The listing builds one solid part. Answer for the finished solid, in the listing's coordinates (mm). A direction names the side the tool comes from. Coordinates: 2 decimals unless noted, no trailing zeros. Loops run counter-clockwise (first coordinate to the right, second up) from the corner with the lowest first, then second, coordinate; pieces in that order, holes last. Notation, with made-up numbers: (-32.75, 86.5) - (-4.75, 86.5) arc R18 cw to (-4.75, 99.5) - close; hole circle Ø9 at (-30.75, -28.75). An arc over 180 degrees is marked (long way). Write each question's results on one line, items separated by ' | '. Start each with the question number.
(1) Find section B-B on z = 11.25. Determine the outline of the cut face in (x, y), then the cut area to 3 significant figures.
(2) Find section A-A on y = 3. Determine the outline of the cut face in (x, z), then the cut area to 3 significant figures.
(3) Find section D-D on x = -19. Determine the outline of the cut face in (y, z), then the cut area to 3 significant figures.
(4) Given pin 1 Ø1.5 at (x, y) = (-1, 2) entering from -Z; pin 2 Ø1.8 at (y, z) = (3.5, 7.5) entering from +X; pin 3 Ø3 at (y, z) = (1.5, 10.5) entering from -X; pin 4 Ø1.8 at (y, z) = (3, 3.1) entering from +X, each flat-ended and moving along its own axis, determine where each tip first touches the part or whether it passes through.
(5) Consider line 1 (Y direction, x = -18.5, z = 3.1); line 2 (Z direction, x = -1.5, y = 3.9); line 3 (X direction, y = 5.05, z = 5.5). Determine where each line is inside the solid, lowest interval first. Write a range as from..to.
(6) For faces 4 (the flat face through (-6.1, 3, 6)), 5 (the flat face through (-11, 0, 10)), 6 (the flat face through (-2, 3, 9)), determine the directions among +Z, -Z, +X, -X, +Y, -Y from which every point of the face is accessible in a straight line to the end or side of a thin tool.
(7) Determine the mould class of faces 1 (the flat face through (-5, 3, 17)), 2 (the flat face through (-3, 3, 11)), 3 (the flat face through (0, 3, 13)) for opening direction X: released by +X, released by -X, zero draft, split by the parting line, or undercut.
(8) Find section C-C on x = -5. Determine the outline of the cut face in (y, z).
Autodesk Inventor part; units mm, degrees
ref_plane "YZ Plane" through (0, 0, 0) normal (1, 0, 0) x (0, 1, 0)
ref_plane "XZ Plane" through (0, 0, 0) normal (0, 1, 0) x (-1, 0, 0)
ref_plane "XY Plane" through (0, 0, 0) normal (0, 0, 1) x (1, 0, 0)
sketch "Sketch1" plane through (0, 0, 0) normal (0, 1, 0) x (-1, 0, 0)
  line L0 (0, 0) -> (21.6, 0)
  line L1 (21.6, 0) -> (21.6, 17)
  line L2 (21.6, 17) -> (0, 17)
  line L3 (0, 17) -> (0, 0)
  line L4 (6.1, 13) -> (3, 13)
  line L5 (3, 13) -> (3, 0)
  line L6 (3, 0) -> (6.1, 0)
  line L7 (6.1, 0) -> (6.1, 13)
  line L8 (21.6, 17) -> (9.1, 17)
  line L9 (9.1, 17) -> (9.1, 0)
  line L10 (9.1, 0) -> (21.6, 0)
  line L11 (21.6, 0) -> (21.6, 17)
  line L12 (9.1, 17) -> (21.6, 6.2)
  point P0 (21.6, 6.2)
  point P1 (9.1, 17)
  dimension "d1" = 17
  dimension "d2" = 3.1
  dimension "d3" = 3
  dimension "d4" = 3
  dimension "d5" = 6.2
  dimension "d17" = 13
  dimension "d18" = 12.5
extrude "Extrusion1" add sketch "Sketch1" along normal blind 6 contours L3 L2 L9 L0 L7 L4 L5 | L12 L1 L0 L9
sketch "Sketch2" plane through (-21.6, 0, 0) normal (-1, 0, 0) x (0, 0, 1)
  circle A0 centre (3.1, 3) radius 3
  line L0 (0, 0) -> (13, 0)
  line L1 (0, 0) -> (0, 6)
  line L2 (17, 6) -> (0, 6)
  line L3 (0, 0) -> (6.2302, 0)
  line L4 (6.2302, 0) -> (6.2302, 6)
  line L5 (6.2302, 6) -> (0, 6)
  line L6 (0, 6) -> (0, 0)
  circle A1 centre (3.1, 3) radius 1
  point P0 (3.1, 6)
  point P1 (3.1, 0)
  dimension "d8" = 3.1
  dimension "d9" = 2
extrude "Extrusion2" cut sketch "Sketch2" against normal up to surface (18.6 mm away) contours A0 L0 L1 L2 | A1
sketch "Sketch3" plane through (0, 6, 0) normal (0, 1, 0) x (1, 0, 0)
  line L0 (-3, 0) -> (-3, -13)
  line L1 (0, 0) -> (-3, 0)
  line L2 (-3, -9) -> (0, -9)
  line L3 (0, -9) -> (0, 0)
  line L4 (0, 0) -> (-3, 0)
  line L5 (-3, 0) -> (-3, -9)
  line L6 (-3, -13) -> (-6.1, -13)
  line L7 (-9.1, -17) -> (0, -17)
  dimension "d13" = 8
extrude "Extrusion3" cut sketch "Sketch3" against normal blind 10
properties part number "Pi3B_spacer_R"
Values:
1) outline: (-15.76, 0) - (-6.1, 0) - (-6.1, 6) - (-15.76, 6) - close; (-3, 0) - (0, 0) - (0, 6) - (-3, 6) - close | area: 75.9 mm²
2) outline: (-21.6, 0.1) - (-6.1, 0.1) - (-6.1, 2.1) - (-21.6, 2.1) - close; (-21.6, 4.1) - (-6.1, 4.1) - (-6.1, 13) - (-3, 13) - (-3, 9) - (0, 9) - (0, 17) - (-9.1, 17) - (-21.6, 6.2) - close | area: 200 mm²
3) outline: (0, 3.1) arc R3 ccw to (6, 3.1) - (6, 8.45) - (0, 8.45) - close; hole circle Ø2 at (3, 3.1) | area: 43.1 mm²
4) pin 1: stops at z = 9 | pin 2: stops at x = -6.1 | pin 3: stops at x = -18.36 | pin 4: passes through
5) line 1: y = 0..2, 4..6 | line 2: z = 9..17 | line 3: x = -21.6..-6.1
6) face 4: -Z, +Y, -Y | face 5: +Z, -Z, +X, -X, -Y | face 6: -Z, +X, +Y, -Y
7) face 1: zero draft | face 2: undercut | face 3: released by +X
8) outline: (0, 13) - (6, 13) - (6, 17) - (0, 17) - close
